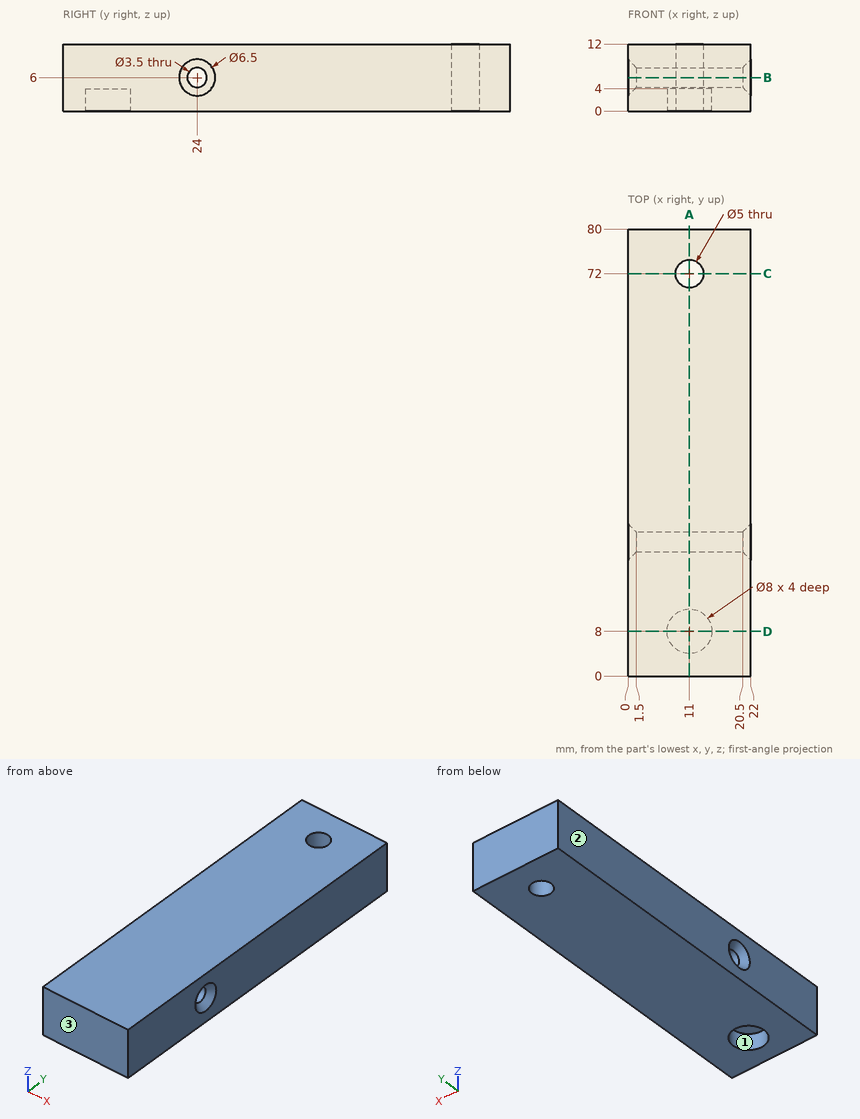
Job drawing, mm, ordinate dimensions from the low corner. One solid piece. Give positions to 0.01 mm unless a question says otherwise; leave off trailing zeros. Loops run counter-clockwise (first coordinate to the right, second up) from the corner with the lowest first, then second, coordinate; pieces in that order, holes last. Notation, with made-up numbers: (10.5, -27.75) -> (56.5, -27.75) arc R18 ccw to (56.5, -5.75) -> close; hole circle Ø3 at (86, 77). An arc over 180 degrees is marked (long way). Use a Markdown table: item, result. Add a question column.
(1) Wall check: line 1 along Y through (x, z) = (11, 2.15); line 2 along Z through (x, y) = (9, 24); line 3 along Y through (x, z) = (12, 1.25). Give the ranges that are in metal, low to high.
(2) Slice it at D-D on y = 8. List the corners of the cut face in (x, z), and give its area (3 significant figures).
(3) Slice it at C-C on y = 72. List the corners of the cut face in (x, z).
(4) Mould opens along Y. For the marked faces 1, 2 and 3 say: +Y half, -Y half, draft (parallel to the pull), parting line (faces both ways), or undercut.
(5) Drop flat-ended pins along their axis: pin 1 Ø2.5 at (x, y) = (10.5, 8) entering from -Z; pin 2 Ø4.5 at (y, z) = (24, 6) entering from -X. Give the stop position or say it passes through.
(6) Slice it at A-A on x = 11. List the corners of the cut face in (y, z).
(7) Slice it at B-B on z = 6. List the corners of the cut face in (x, y).
Filled sheet:
| question | item | result |
|---|---|---|
| 1 | line 1 | 0 to 4, 12 to 69.5, 74.5 to 80 |
| 1 | line 2 | 0 to 4.25, 7.75 to 12 |
| 1 | line 3 | 0 to 4.13, 11.87 to 69.71, 74.29 to 80 |
| 2 | outline | (0, 0) -> (7, 0) -> (7, 4) -> (15, 4) -> (15, 0) -> (22, 0) -> (22, 12) -> (0, 12) -> close |
| 2 | area | 232 mm2 |
| 3 | outline | (0, 0) -> (8.5, 0) -> (8.5, 12) -> (0, 12) -> close; (13.5, 0) -> (22, 0) -> (22, 12) -> (13.5, 12) -> close |
| 4 | face 1 | undercut |
| 4 | face 2 | draft |
| 4 | face 3 | -Y half |
| 5 | pin 1 | z = 4 |
| 5 | pin 2 | x = 1 |
| 6 | outline | (0, 0) -> (4, 0) -> (4, 4) -> (12, 4) -> (12, 0) -> (69.5, 0) -> (69.5, 12) -> (0, 12) -> close; (74.5, 0) -> (80, 0) -> (80, 12) -> (74.5, 12) -> close; hole circle Ø3.5 at (24, 6) |
| 7 | outline | (0, 0) -> (22, 0) -> (22, 20.75) -> (20.5, 22.25) -> (1.5, 22.25) -> (0, 20.75) -> close; (0, 27.25) -> (1.5, 25.75) -> (20.5, 25.75) -> (22, 27.25) -> (22, 80) -> (0, 80) -> close; hole circle Ø5 at (11, 72) |
